Autodesk Inventor part; units mm, degrees
ref_plane "Work Plane1" through (8, 0, 0) normal (0, 0.5, 0.866) x (1, 0, 0)
ref_plane "YZ Plane" through (0, 0, 0) normal (1, 0, 0) x (0, 1, 0)
ref_plane "XZ Plane" through (0, 0, 0) normal (0, 1, 0) x (-1, 0, 0)
sketch "Эскиз1" plane through (0, 0, 0) normal (0, 0, 1) x (1, 0, 0)
  line L0 (1.0774, 0) -> (16, 0)
  line L1 (16, 0) -> (16, 2)
  line L2 (16, 2) -> (0, 2)
  line L3 (0, 2) -> (0, 3.5)
  line L4 (0, 3.5) -> (-2.8, 3.5)
  line L5 (-2.8, 3.5) -> (-2.8, 1.7321)
  line L6 (-2.8, 1.7321) -> (-1.2, 1.7321)
  line L7 (-1.2, 1.7321) -> (-0.7774, 1)
  line L8 (-6.56, 0) -> (19.76, 0)
  line L9 (0, -0.7) -> (0, 4.2)
  line L10 (-0.7774, 1) -> (0.5, 1)
  line L11 (0.5, 1) -> (1.0774, 0)
  line L12 (-2.8, 1.7321) -> (-2.8, 0) construction
  line L13 (-2.8, 3.1) -> (-2.4, 3.5)
  dimension "d0" = 2.8
  dimension "d1" = 1.6
  dimension "d2" = 60
  dimension "d3" = 4
  dimension "d4" = 3.4641
  dimension "d5" = 7
  dimension "d15" = 3.3
  dimension "d16" = 2
  dimension "d17" = 16
  dimension "d32" = 45
  dimension "d33" = 0.4
revolve "Базовый элемент" add sketch "Эскиз1" angle 360 about axis through (1.0774, 0, 0) along (1, 0, 0) contours L11 L10 L9 L2 L1 L0 | L10 L7 L6 L5 L13 L4 L3 L9 | L13 L5 L4
revolve "Фаска2" cut sketch "Эскиз1" angle 360 about axis through (-10, 0, 0) along (1, 0, 0) contours L13 L5 L4
sketch "Эскиз2" plane through (-2.8, 0, 0) normal (-1, 0, 0) x (0, 0, 1)
  circle A0 centre (0, 0) radius 1.7321
  line L0 (0, -4.9) -> (0, 4.9)
  line L1 (-4.9, 0) -> (4.9, 0)
  line L2 (1.7321, 0) -> (0.866, -1.5)
  line L3 (0.866, -1.5) -> (-0.866, -1.5)
  line L4 (-0.866, -1.5) -> (-1.7321, 0)
  line L5 (-1.7321, 0) -> (-0.866, 1.5)
  line L6 (-0.866, 1.5) -> (0.866, 1.5)
  line L7 (0.866, 1.5) -> (1.7321, 0)
extrude "Паз" add sketch "Эскиз2" against normal up to next contours L7 A0 | A0 L2 | L6 L0 A0 | A0 L0 L3 | L0 L6 A0 | A0 L3 L0 | L4 A0 | A0 L5
thread "Резьба"
chamfer "Фаска1" distance 0.4294 distance2 0.4294 1 edges at (16, -2, 0) measured on face at (16, 0.527, -0.2661)
ref_plane "Work Plane1" through (8, 0, 0) normal (0, 0.5, 0.866) x (1, 0, 0)
equation "\"d0\" = KOH"
equation "\"d1\" = INTI"
equation "\"d3\" = GD"
equation "\"d4\" = 1.1547 * SW"
equation "\"d5\" = KOD"
equation "\"d15\" = INFT"
equation "\"d16\" = SDT"
equation "\"d17\" = NLG"
equation "\"d33\" = Cham"
equation "\"d7\" = GEL"
equation "\"d9\" = -0.5 * SPD + 0.5 * GD"
equation "\"d12\" = GUL"
equation "\"GD\" = NND"
equation "\"NLG\" = 16"
equation "\"GEL\" = 12.5"
equation "\"KOD\" = 7"
equation "\"KOH\" = 2.8"
equation "\"GUL\" = 0.61345 * PTC"
equation "\"SW\" = 3"
equation "\"INTI\" = 1.6"
equation "\"SPD\" = NND - 1.2269 * PTC"
equation "\"SDT\" = 2"
equation "\"INFT\" = 3.3"
equation "\"Cham\" = 0.4"
equation "\"TOA\" = 30deg"
equation "\"GD1\" = THREADDIA - 1.2269 * PTC"
equation "\"THREADDIA\" = 4"
equation "\"BDM\" = NND"
equation "\"FAWI\" = 45deg"
equation "\"RR\" = 0.1 * NND"
equation "\"PTC\" = 0.7"
equation "\"NND\" = 4"
equation "\"FAWI1\" = 45deg"
equation "\"GAL\" = 0.61345 * PTC"
equation "\"E0\" = 1.155 * SW"
properties part number "DIN 6912 - M4 x 16" material "Сталь, мягкая"
Can you work these out from the model? Positions are in its coordinate system, mm. A direction names the side the tool comes from. Coordinates: 2 decimals unless noted, no trailing zeros. Loops run counter-clockwise (first coordinate to the right, second up) from the corner with the lowest first, then second, coordinate; pieces in that order, holes last. Notation, with made-up numbers: (43, 68) -> (77, 68) arc R14 cw to (77, 72) -> close; hole circle Ø4 at (60, 20). An arc over 180 degrees is marked (long way). Put each result on its own line as item: value. Start each with the question number.
Q1. I want a section at A-A (x = 5.5). Write out the boundary of the cut face in (y, z), plus the area to 3 significant figures.
Q2. I'm going to push flat-ended pins straight in: P1, Ø3, axis at x = 5.5, y = 2.5, coming from the +Z side; P2, Ø2, axis at y = -2.5, z = -2.5, coming from the +X side; P3, Ø1.5, axis at x = 11.5, z = 1.5, coming from the +Y side. Where does each tip first touch, or does it pass through?
Q3. For faces 1 (the face through (8, 0, 2)), 2 (the face through (-1.945, -0.761, -1.293)), 3 (the face through (-1.217, 3.233, 1.341)), which set-ups out of +Z, -Z, +X, -X, +Y, -Y let a thin tool reach every point of the face, with its end or its side?
Q4. If I drill on line 1 (Z direction, x = 0.05, y = 0); line 2 (X direction, y = -3, z = -0.25); line 3 (Z direction, x = -0.2, y = 0), over which ranges is the centre line in solid material (lowest first)? Write a range as [from, to].
Taken from the geometry:
1. outline: circle Ø4 at (0, 0)
1. area: 12.6 mm2
2. P1: stops at z = 1.73
2. P2: stops at x = 0
2. P3: stops at y = 1.85
3. face 1: +X
3. face 2: -X
3. face 3: +X, -X
4. line 1: z = [-2, -1], [1, 2]
4. line 2: x = [-2.8, 0]
4. line 3: z = [-3.5, -1], [1, 3.5]
